Check sheet for the modelled part. Datum: model origin and axes. Units: mm. Give positions to 0.01 mm unless a question says otherwise; leave off trailing zeros. Write each loop counter-clockwise with the first axis right and the second up, starting at its lowest first coordinate (ties: lowest second). Pieces come first, ordered by that corner, then holes. Notation, with made-up numbers: (-28.5, -29) -> (-17.5, -29) arc R17 cw to (-17.5, -6) -> close; hole circle Ø8 at (76.25, -22.5). An arc over 180 degrees is marked (long way). Use a Markdown table: item, result. Add a question column.
1. Gauge pin test, flat ends, axial feed: P1, Ø1.9, axis at x = 42.5, y = -30.1, coming from the +Z side; P2, Ø3.5, axis at x = -42.5, y = 30.1, coming from the +Z side. Record the tip position at first contact, or that the pin passes through.
2. Cross-section at B-B (x = -24). Enter the section's corners in (y, z), then the cut area to 3 significant figures.
3. Cross-section at A-A (y = -3). Enter the section's corners in (x, z).
4. Cross-section at D-D (z = 1.55). Count the separate pieces of the cut face and the enclosed holes in it, then the cut area to 3 significant figures.
5. Cross-section at C-C (y = 10). Enter the section's corners in (x, z), then the cut area to 3 significant figures.
6. Release check for a two-part mould opening along X. For faces 1 (the flat face through (0, 0, 0)), 2 (the cylindrical face through (46, -33.67, 1.48)), 3 (the cylindrical face through (-41.25, -25.26, 1.48)) record: released by +X, released by -X, zero draft, split by the parting line, or undercut.
7. Scan lines: probe 1 along Y at (x, z) = (42.5, 1.6); probe 2 along X at (y, z) = (-6.5, 0.7); probe 3 along X at (y, z) = (20.5, 0.6). Record each from-to range of solid material in increasing order. Write a range as [from, to].
from build123d import *

# Parameters (mm, degrees)
SKETCH_1_R      = 5
SKETCH_1_R_2    = 1.55
EXTRUDE_1_DEPTH = 3
FILLET_1_R      = 2
FILLET_2_R      = 1


with BuildPart() as part:
    # 草图1 → 凸台-拉伸1 (new body)
    # profile 1 of 5: a face of its own
    with BuildSketch(Plane.XY):
        with BuildLine():
            Line((-42.5, -35.1), (42.5, -35.1))
            ThreePointArc((42.5, -35.1), (39.761387212, -34.283300133), (37.917424305, -32.1))
            Line((37.917424305, -32.1), (2, -32.1))
            Line((2, -32.1), (2, -3.964694458))
            Line((2, -3.964694458), (37.500961204, -30.198036316))
            ThreePointArc((37.500961204, -30.198036316), (37.902514018, -28.134517198), (39.116783888, -26.418444794))
            Line((39.116783888, -26.418444794), (6.071879965, -2))
            Line((6.071879965, -2), (44.5, -2))
            Line((44.5, -2), (44.5, -25.517424305))
            ThreePointArc((44.5, -25.517424305), (46.683300133, -27.361387212), (47.5, -30.1))
            Line((47.5, -30.1), (47.5, 30.1))
            ThreePointArc((47.5, 30.1), (46.683300133, 27.361387212), (44.5, 25.517424305))
            Line((44.5, 25.517424305), (44.5, 2))
            Line((44.5, 2), (6.071879965, 2))
            Line((6.071879965, 2), (39.116783888, 26.418444794))
            ThreePointArc((39.116783888, 26.418444794), (37.902514018, 28.134517198), (37.500961204, 30.198036316))
            Line((37.500961204, 30.198036316), (2, 3.964694458))
            Line((2, 3.964694458), (2, 32.1))
            Line((2, 32.1), (37.917424305, 32.1))
            ThreePointArc((37.917424305, 32.1), (39.761387212, 34.283300133), (42.5, 35.1))
            Line((42.5, 35.1), (-42.5, 35.1))
            ThreePointArc((-42.5, 35.1), (-39.761387212, 34.283300133), (-37.917424305, 32.1))
            Line((-37.917424305, 32.1), (-2, 32.1))
            Line((-2, 32.1), (-2, 3.964694458))
            Line((-2, 3.964694458), (-37.500961204, 30.198036316))
            ThreePointArc((-37.500961204, 30.198036316), (-37.500240307, 30.149020514), (-37.5, 30.1))
            ThreePointArc((-37.5, 30.1), (-37.922004775, 28.089537437), (-39.116783888, 26.418444794))
            Line((-39.116783888, 26.418444794), (-6.071879965, 2))
            Line((-6.071879965, 2), (-44.5, 2))
            Line((-44.5, 2), (-44.5, 25.517424305))
            ThreePointArc((-44.5, 25.517424305), (-46.683300133, 27.361387212), (-47.5, 30.1))
            Line((-47.5, 30.1), (-47.5, -30.1))
            ThreePointArc((-47.5, -30.1), (-46.683300133, -27.361387212), (-44.5, -25.517424305))
            Line((-44.5, -25.517424305), (-44.5, -2))
            Line((-44.5, -2), (-6.071879965, -2))
            Line((-6.071879965, -2), (-39.116783888, -26.418444794))
            ThreePointArc((-39.116783888, -26.418444794), (-37.922004775, -28.089537437), (-37.5, -30.1))
            ThreePointArc((-37.5, -30.1), (-37.500240307, -30.149020514), (-37.500961204, -30.198036316))
            Line((-37.500961204, -30.198036316), (-2, -3.964694458))
            Line((-2, -3.964694458), (-2, -32.1))
            Line((-2, -32.1), (-37.917424305, -32.1))
            ThreePointArc((-37.917424305, -32.1), (-39.761387212, -34.283300133), (-42.5, -35.1))
        make_face()
    # profile 2 of 5: a face of its own
    with BuildSketch(Plane.XY):
        with Locations((-42.5, 30.1)):
            Circle(SKETCH_1_R)
        with Locations((-42.5, 30.1)):
            Circle(SKETCH_1_R_2, mode=Mode.SUBTRACT)
    # profile 3 of 5: a face of its own
    with BuildSketch(Plane.XY):
        with Locations((42.5, 30.1)):
            Circle(SKETCH_1_R)
        with Locations((42.5, 30.1)):
            Circle(SKETCH_1_R_2, mode=Mode.SUBTRACT)
    # profile 4 of 5: a face of its own
    with BuildSketch(Plane.XY):
        with Locations((42.5, -30.1)):
            Circle(SKETCH_1_R)
        with Locations((42.5, -30.1)):
            Circle(SKETCH_1_R_2, mode=Mode.SUBTRACT)
    # profile 5 of 5: a face of its own
    with BuildSketch(Plane.XY):
        with Locations((-42.5, -30.1)):
            Circle(SKETCH_1_R)
        with Locations((-42.5, -30.1)):
            Circle(SKETCH_1_R_2, mode=Mode.SUBTRACT)
    extrude(amount=EXTRUDE_1_DEPTH)

    # 圆角1
    # the kernel refuses this fillet: 2 mm, written as the material it adds along each edge
    with BuildSketch(Plane(origin=(39.116783888, 26.418444794, 0), x_dir=(-0.8042465112804378, -0.5942958430724927, 0), z_dir=(0, 0, 1)), Plane(origin=(-39.116783888, -26.418444794, 0), x_dir=(0.8042465112804382, 0.5942958430724918, 0), z_dir=(0, 0, 1))) as fillet_1_piece_1:
        with BuildLine():
            CenterArc((1.439043849, 2), FILLET_1_R, 204.927038376, 65.072961624)
            ThreePointArc((-0.374646596, 1.157072383), (-0.152011037, 0.589969891), (0, 0))
            Line((0, 0), (1.439043849, 0))
        make_face()
    extrude(amount=3)
    with BuildSketch(Plane(origin=(6.071879965, 2, 0), x_dir=(1, 0, 0), z_dir=(0, 0, 1)), Plane(origin=(6.071879965, -2, 0), x_dir=(0.804246511280438, -0.5942958430724921, 0), z_dir=(0, 0, 1)), Plane(origin=(-6.071879965, -2, 0), x_dir=(-1, 0, 0), z_dir=(0, 0, 1)), Plane(origin=(-6.071879965, 2, 0), x_dir=(-0.8042465112804379, 0.5942958430724924, 0), z_dir=(0, 0, 1))) as fillet_1_piece_2:
        with BuildLine():
            CenterArc((FILLET_1_R * 3.03593998227, FILLET_1_R), FILLET_1_R, 126.462450613, 143.537549387)
            Line((FILLET_1_R * 2.4416441392, FILLET_1_R * 1.80424651128), (0, 0))
            Line((0, 0), (FILLET_1_R * 3.03593998227, 0))
        make_face()
    extrude(amount=3)
    with BuildSketch(Plane(origin=(44.5, 2, 0), x_dir=(0, 1, 0), z_dir=(0, 0, 1)), Plane(origin=(44.5, -2, 0), x_dir=(-1, 0, 0), z_dir=(0, 0, 1)), Plane(origin=(2, -32.1, 0), x_dir=(1, 0, 0), z_dir=(0, 0, 1)), Plane(origin=(-2, -32.1, 0), x_dir=(0, 1, 0), z_dir=(0, 0, 1)), Plane(origin=(-44.5, -2, 0), x_dir=(0, -1, 0), z_dir=(0, 0, 1)), Plane(origin=(-44.5, 2, 0), x_dir=(1, 0, 0), z_dir=(0, 0, 1)), Plane(origin=(-2, 32.1, 0), x_dir=(-1, 0, 0), z_dir=(0, 0, 1)), Plane(origin=(2, 32.1, 0), x_dir=(0, -1, 0), z_dir=(0, 0, 1))) as fillet_1_piece_3:
        with BuildLine():
            CenterArc((FILLET_1_R, FILLET_1_R), FILLET_1_R, 180, 90)
            Line((0, FILLET_1_R), (0, 0))
            Line((0, 0), (FILLET_1_R, 0))
        make_face()
    extrude(amount=3)
    with BuildSketch(Plane(origin=(44.5, 25.517424305, 0), x_dir=(0, -1, 0), z_dir=(0, 0, 1)), Plane(origin=(37.917424305, -32.1, 0), x_dir=(-1, 0, 0), z_dir=(0, 0, 1)), Plane(origin=(-44.5, -25.517424305, 0), x_dir=(0, 1, 0), z_dir=(0, 0, 1)), Plane(origin=(-37.917424305, 32.1, 0), x_dir=(1, 0, 0), z_dir=(0, 0, 1))) as fillet_1_piece_4:
        with BuildLine():
            CenterArc((2.417424305, -2), FILLET_1_R, 90, 90)
            ThreePointArc((0.417424305, -2), (0.31195587, -0.978451782), (0, 0))
            Line((0, 0), (2.417424305, 0))
        make_face()
    extrude(amount=3)
    with BuildSketch(Plane(origin=(44.5, -25.517424305, 0), x_dir=(0, 1, 0), z_dir=(0, 0, 1)), Plane(origin=(-37.917424305, -32.1, 0), x_dir=(1, 0, 0), z_dir=(0, 0, 1)), Plane(origin=(-44.5, 25.517424305, 0), x_dir=(0, -1, 0), z_dir=(0, 0, 1)), Plane(origin=(37.917424305, 32.1, 0), x_dir=(-1, 0, 0), z_dir=(0, 0, 1))) as fillet_1_piece_5:
        with BuildLine():
            CenterArc((2.417424305, 2), FILLET_1_R, 180, 90)
            ThreePointArc((0.417424305, 2), (0.31195587, 0.978451782), (0, 0))
            Line((0, 0), (2.417424305, 0))
        make_face()
    extrude(amount=3)
    with BuildSketch(Plane(origin=(39.116783888, -26.418444794, 0), x_dir=(-0.8042465112804377, 0.5942958430724928, 0), z_dir=(0, 0, 1)), Plane(origin=(-39.116783888, 26.418444794, 0), x_dir=(0.8042465112804396, -0.5942958430724902, 0), z_dir=(0, 0, 1))) as fillet_1_piece_6:
        with BuildLine():
            CenterArc((1.439043849, -2), FILLET_1_R, 90, 65.072961624)
            ThreePointArc((-0.374646596, -1.157072383), (-0.152011037, -0.589969891), (0, 0))
            Line((0, 0), (1.439043849, 0))
        make_face()
    extrude(amount=3)
    with BuildSketch(Plane(origin=(2, -3.964694458, 0), x_dir=(0, -1, 0), z_dir=(0, 0, 1)), Plane(origin=(-2, -3.964694458, 0), x_dir=(-0.8042465112804379, -0.5942958430724925, 0), z_dir=(0, 0, 1)), Plane(origin=(-2, 3.964694458, 0), x_dir=(0, 1, 0), z_dir=(0, 0, 1)), Plane(origin=(2, 3.964694458, 0), x_dir=(0.804246511280438, 0.5942958430724923, 0), z_dir=(0, 0, 1))) as fillet_1_piece_7:
        with BuildLine():
            CenterArc((FILLET_1_R * 1.982347229, FILLET_1_R), FILLET_1_R, 143.537549387, 126.462450613)
            Line((FILLET_1_R * 1.17810071772, FILLET_1_R * 1.59429584307), (0, 0))
            Line((0, 0), (FILLET_1_R * 1.982347229, 0))
        make_face()
    extrude(amount=3)
    with BuildSketch(Plane(origin=(37.500961204, -30.198036316, 0), x_dir=(-0.8042465112804396, 0.5942958430724902, 0), z_dir=(0, 0, 1)), Plane(origin=(-37.500961204, 30.198036316, 0), x_dir=(0.8042465112804383, -0.5942958430724916, 0), z_dir=(0, 0, 1))) as fillet_1_piece_8:
        with BuildLine():
            CenterArc((0.885482013, 2), FILLET_1_R, 226.169636842, 43.830363158)
            ThreePointArc((-0.499569115, 0.557213331), (-0.239344892, 0.287966338), (0, 0))
            Line((0, 0), (0.885482013, 0))
        make_face()
    extrude(amount=3)
    with BuildSketch(Plane(origin=(-37.500961204, -30.198036316, 0), x_dir=(0.8042465112804397, 0.59429584307249, 0), z_dir=(0, 0, 1)), Plane(origin=(37.500961204, 30.198036316, 0), x_dir=(-0.8042465112804407, -0.5942958430724886, 0), z_dir=(0, 0, 1))) as fillet_1_piece_9:
        with BuildLine():
            CenterArc((0.885482013, -2), FILLET_1_R, 90, 43.830363158)
            ThreePointArc((-0.499569115, -0.557213331), (-0.239344892, -0.287966338), (0, 0))
            Line((0, 0), (0.885482013, 0))
        make_face()
    extrude(amount=3)

    # 圆角2
    fillet_2_edges = [part.edges().sort_by_distance(p)[0] for p in [
        (37.453554234, -30.528515876, 1.5),
        (-37.453554234, -30.528515876, 1.5),
        (-37.453554234, 30.528515876, 1.5),
        (37.453554234, 30.528515876, 1.5),
    ]]
    fillet(fillet_2_edges, radius=FILLET_2_R)


solid = part.part
Worked answers:
| question | item | result |
|---|---|---|
| 1 | P1 | passes through |
| 1 | P2 | stops at z = 3 |
| 2 | outline | (-35.1, 0) -> (-32.1, 0) -> (-32.1, 3) -> (-35.1, 3) -> close; (-20.22, 0) -> (-15.25, 0) -> (-15.25, 3) -> (-20.22, 3) -> close; (-2, 0) -> (2, 0) -> (2, 3) -> (-2, 3) -> close; (15.25, 0) -> (20.22, 0) -> (20.22, 3) -> (15.25, 3) -> close; (32.1, 0) -> (35.1, 0) -> (35.1, 3) -> (32.1, 3) -> close |
| 2 | area | 59.8 mm² |
| 3 | outline | (-47.5, 0) -> (-44.23, 0) -> (-44.23, 3) -> (-47.5, 3) -> close; (-10.41, 0) -> (10.41, 0) -> (10.41, 3) -> (-10.41, 3) -> close; (44.23, 0) -> (47.5, 0) -> (47.5, 3) -> (44.23, 3) -> close |
| 4 | separate pieces | 1 |
| 4 | enclosed holes | 12 |
| 4 | area | 2,430 mm² |
| 5 | outline | (-47.5, 0) -> (-44.5, 0) -> (-44.5, 3) -> (-47.5, 3) -> close; (-16.9, 0) -> (-10.17, 0) -> (-10.17, 3) -> (-16.9, 3) -> close; (-2, 0) -> (2, 0) -> (2, 3) -> (-2, 3) -> close; (10.17, 0) -> (16.9, 0) -> (16.9, 3) -> (10.17, 3) -> close; (44.5, 0) -> (47.5, 0) -> (47.5, 3) -> (44.5, 3) -> close |
| 5 | area | 70.4 mm² |
| 6 | face 1 | zero draft |
| 6 | face 2 | released by +X |
| 6 | face 3 | undercut |
| 7 | probe 1 | y = [-35.1, -31.65], [-28.55, -25.1], [-2, 2], [25.1, 28.55], [31.65, 35.1] |
| 7 | probe 2 | x = [-47.5, -44.5], [-12.16, -5.43], [-2.6, 2.6], [5.43, 12.16], [44.5, 47.5] |
| 7 | probe 3 | x = [-47.5, -44.5], [-31.11, -24.38], [-2, 2], [24.38, 31.11], [44.5, 47.5] |
